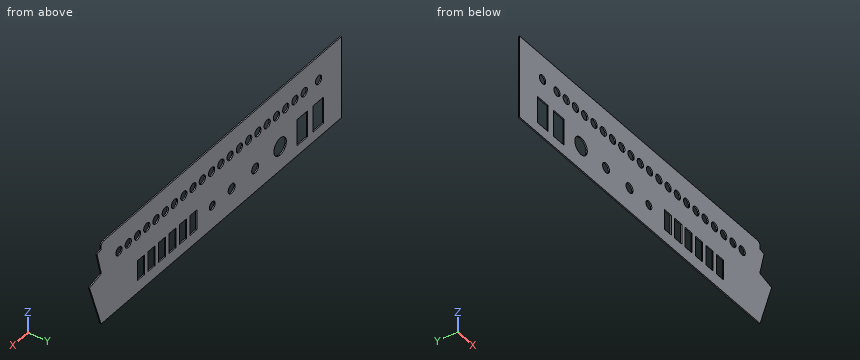
from build123d import *

# Parameters (mm, degrees)
SKETCH4_R           = 11.95
SKETCH4_R_2         = 6.65
SKETCH4_R_3         = 5.6
SKETCH4_R_4         = 6
SKETCH4_W           = 20.218579234
SKETCH4_H           = 37
SKETCH4_W_2         = 13.5
SKETCH4_H_2         = 28.1
BOSS_EXTRUDE3_DEPTH = 1.6


with BuildPart() as part:
    # Sketch4 → Boss-Extrude3 (new body)
    with BuildSketch(Plane(origin=(0, 0, 0), x_dir=(1, 0, 0), z_dir=(0, 1, 0))):
        with BuildLine():
            Line((-63.047420146, 63.390203379), (-63.047420146, -51.609796621))
            Line((-63.047420146, -51.609796621), (392.952579854, -51.609796621))
            ThreePointArc((392.952579854, -51.609796621), (396.48811376, -50.145330527), (397.952579854, -46.609796621))
            Line((397.952579854, -46.609796621), (397.952579854, -42.187494758))
            Line((397.952579854, -42.187494758), (405.679986464, -40.116942397))
            Line((405.679986464, -40.116942397), (397.952579854, -9.609796621))
            Line((397.952579854, -9.609796621), (397.952579854, -7.609796621))
            Line((397.952579854, -7.609796621), (420.168873859, -1.656958583))
            Line((420.168873859, -1.656958583), (397.952579854, 63.390203379))
            Line((397.952579854, 63.390203379), (-63.047420146, 63.390203379))
        make_face()
        with Locations(Location((54.9, 29.690203379, 0), (0, 0, 270))):
            Circle(SKETCH4_R, mode=Mode.SUBTRACT)
        with Locations(Location((102.75, 30.240203379, 0), (0, 0, 270))):
            Circle(SKETCH4_R_2, mode=Mode.SUBTRACT)
        with Locations(Location((147.75, 30.240203379, 0), (0, 0, 270))):
            Circle(SKETCH4_R_2, mode=Mode.SUBTRACT)
        with Locations(Location((184.9, 30.790203379, 0), (0, 0, 270))):
            Circle(SKETCH4_R_3, mode=Mode.SUBTRACT)
        with Locations(Location((-18.9, -18.109796621, 0), (0, 0, 270))):
            Circle(SKETCH4_R_4, mode=Mode.SUBTRACT)
        with Locations(Location((8.7, -18.109796621, 0), (0, 0, 270))):
            Circle(SKETCH4_R_4, mode=Mode.SUBTRACT)
        with Locations(Location((26.45, -18.109796621, 0), (0, 0, 270))):
            Circle(SKETCH4_R_4, mode=Mode.SUBTRACT)
        with Locations(Location((44.2, -18.109796621, 0), (0, 0, 270))):
            Circle(SKETCH4_R_4, mode=Mode.SUBTRACT)
        with Locations(Location((61.95, -18.109796621, 0), (0, 0, 270))):
            Circle(SKETCH4_R_4, mode=Mode.SUBTRACT)
        with Locations(Location((79.7, -18.109796621, 0), (0, 0, 270))):
            Circle(SKETCH4_R_4, mode=Mode.SUBTRACT)
        with Locations(Location((97.45, -18.109796621, 0), (0, 0, 270))):
            Circle(SKETCH4_R_4, mode=Mode.SUBTRACT)
        with Locations(Location((115.2, -18.109796621, 0), (0, 0, 270))):
            Circle(SKETCH4_R_4, mode=Mode.SUBTRACT)
        with Locations(Location((132.95, -18.109796621, 0), (0, 0, 270))):
            Circle(SKETCH4_R_4, mode=Mode.SUBTRACT)
        with Locations(Location((150.7, -18.109796621, 0), (0, 0, 270))):
            Circle(SKETCH4_R_4, mode=Mode.SUBTRACT)
        with Locations(Location((168.45, -18.109796621, 0), (0, 0, 270))):
            Circle(SKETCH4_R_4, mode=Mode.SUBTRACT)
        with Locations(Location((186.2, -18.109796621, 0), (0, 0, 270))):
            Circle(SKETCH4_R_4, mode=Mode.SUBTRACT)
        with Locations(Location((203.95, -18.109796621, 0), (0, 0, 270))):
            Circle(SKETCH4_R_4, mode=Mode.SUBTRACT)
        with Locations(Location((221.7, -18.109796621, 0), (0, 0, 270))):
            Circle(SKETCH4_R_4, mode=Mode.SUBTRACT)
        with Locations(Location((239.45, -18.109796621, 0), (0, 0, 270))):
            Circle(SKETCH4_R_4, mode=Mode.SUBTRACT)
        with Locations(Location((257.2, -18.109796621, 0), (0, 0, 270))):
            Circle(SKETCH4_R_4, mode=Mode.SUBTRACT)
        with Locations(Location((274.95, -18.109796621, 0), (0, 0, 270))):
            Circle(SKETCH4_R_4, mode=Mode.SUBTRACT)
        with Locations(Location((292.7, -18.109796621, 0), (0, 0, 270))):
            Circle(SKETCH4_R_4, mode=Mode.SUBTRACT)
        with Locations(Location((310.45, -18.109796621, 0), (0, 0, 270))):
            Circle(SKETCH4_R_4, mode=Mode.SUBTRACT)
        with Locations(Location((328.2, -18.109796621, 0), (0, 0, 270))):
            Circle(SKETCH4_R_4, mode=Mode.SUBTRACT)
        with Locations(Location((345.95, -18.109796621, 0), (0, 0, 270))):
            Circle(SKETCH4_R_4, mode=Mode.SUBTRACT)
        with Locations(Location((363.7, -18.109796621, 0), (0, 0, 270))):
            Circle(SKETCH4_R_4, mode=Mode.SUBTRACT)
        with Locations((-18.6, 30.690203379)):
            Rectangle(SKETCH4_W, SKETCH4_H, mode=Mode.SUBTRACT)
        with Locations((12.4, 30.690203379)):
            Rectangle(SKETCH4_W, SKETCH4_H, mode=Mode.SUBTRACT)
        with Locations((241.15, 32.073143277)):
            Rectangle(SKETCH4_W_2, SKETCH4_H_2, mode=Mode.SUBTRACT)
        with Locations((221.15, 32.073143277)):
            Rectangle(SKETCH4_W_2, SKETCH4_H_2, mode=Mode.SUBTRACT)
        with Locations((261.15, 32.073143277)):
            Rectangle(SKETCH4_W_2, SKETCH4_H_2, mode=Mode.SUBTRACT)
        with Locations((281.15, 32.073143277)):
            Rectangle(SKETCH4_W_2, SKETCH4_H_2, mode=Mode.SUBTRACT)
        with Locations((301.15, 32.073143277)):
            Rectangle(SKETCH4_W_2, SKETCH4_H_2, mode=Mode.SUBTRACT)
        with Locations((321.15, 32.073143277)):
            Rectangle(SKETCH4_W_2, SKETCH4_H_2, mode=Mode.SUBTRACT)
    extrude(amount=BOSS_EXTRUDE3_DEPTH)


solid = part.part
Could you check a few things on this model? Use its own coordinates, in mm. Coordinates: 2 decimals unless noted, no trailing zeros. Order: outer loops, then holes, each group sorted by start corner. A loop starts at its lowest first (then second) coordinate and runs counter-clockwise, first axis right, second up.
Q1. Please list where these lines run through material, in increasing order: L1, parallel to X at y = 0.1, z = -16; L2, parallel to Z at x = 260.5, y = 0.15; L3, parallel to Z at x = 310.45, y = 1.05.
Q2. Suppose I cut it at B-B on y = 0.3. Give the number of separate pieces and of enclosed holes in the cut face, and give its area (3 significant figures).
Q3. Suppose I cut it at A-A on x = 239.45. Please give me the cut outline in (y, z).
Q4. Will this pin go through, and if not, where does the flat tip stop? pin 1 (0.5 mm diameter, centred on y = 0.5, z = 9, fed in from +X).
Q5. Suppose I cut it at C-C on z = -55. Please give me the cut outline in (x, y).
Answer:
1. L1: x = -63.05 to -28.71, -8.49 to 2.29, 22.51 to 414.14
1. L2: z = -63.39 to -46.12, -18.02 to 13.1, 23.12 to 51.61
1. L3: z = -63.39 to 12.11, 24.11 to 51.61
2. separate pieces: 1
2. enclosed holes: 34
2. area: 46,800 mm2
3. outline: (0, -63.39) - (1.6, -63.39) - (1.6, -46.12) - (0, -46.12) - close; (0, -18.02) - (1.6, -18.02) - (1.6, 12.11) - (0, 12.11) - close; (0, 24.11) - (1.6, 24.11) - (1.6, 51.61) - (0, 51.61) - close
4. pin 1: stops at x = 397.95
5. outline: (-63.05, 0) - (400.82, 0) - (400.82, 1.6) - (-63.05, 1.6) - close
